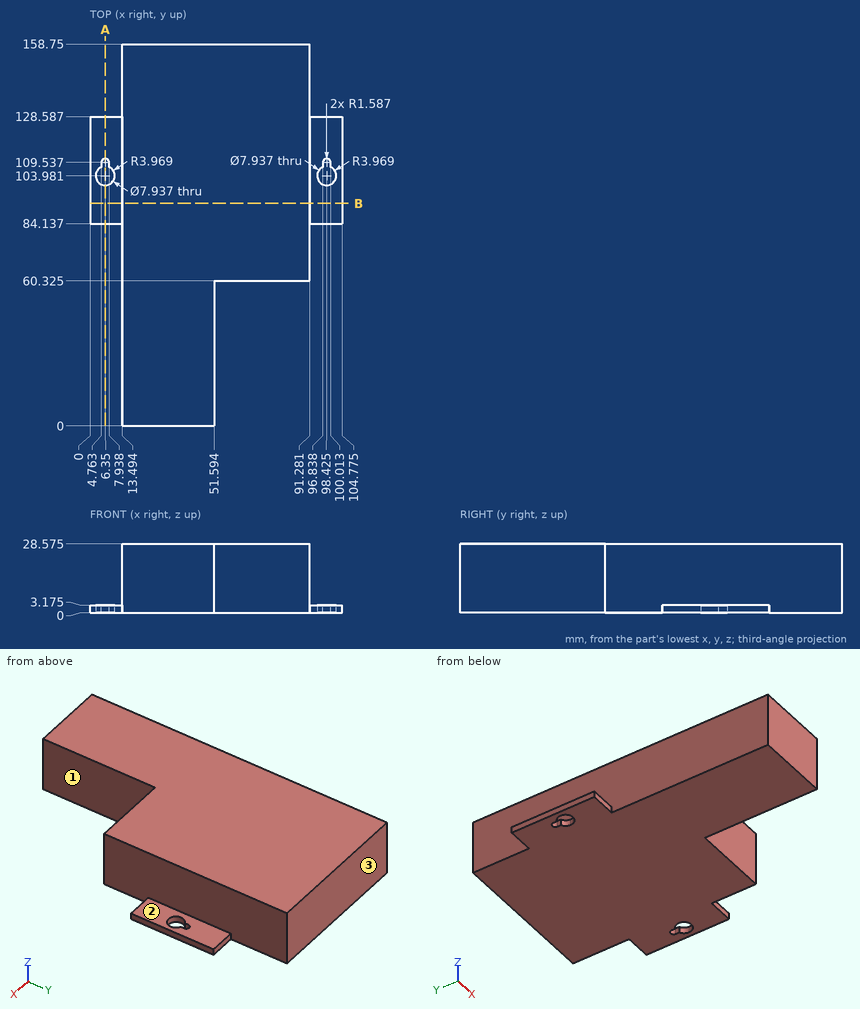
Could you check a few things on this drawing? It's one solid part, dimensions in mm from its lowest x, y, z. A direction names the side the tool comes from. Give positions to 0.01 mm unless a question says otherwise; leave off trailing zeros. Order: outer loops, then holes, each group sorted by start corner. A loop starts at its lowest first (then second) coordinate and runs counter-clockwise, first axis right, second up. Notation, with made-up numbers: (63.5, 53.25) - (115.5, 53.25) arc R13 ccw to (115.5, 62.25) - close; hole circle Ø11 at (79, -6). An arc over 180 degrees is marked (long way). Answer as a JSON object with one key per item and string values. Group by question number.
Item 1: Please list where these lines run through material, in increasing order: probe 1 along Y at (x, z) = (6.35, 1.5) (1 decimal); probe 2 along X at (y, z) = (128.5, 7.75); probe 3 along X at (y, z) = (34, 14.75).
Item 2: For P1, Ø10, axis at y = 55, z = 25, coming from the -X side; P2, Ø12.5, axis at x = 98.43, y = 103.98, coming from the +Z side (1 decimal); P3, Ø0.6, axis at y = 108, z = 2, coming from the -X side; P4, Ø1, axis at x = 96.5, z = 1.5, coming from the +Y side, each with a flat end and sliding along its axis, tell me the tip position at first contact or that it passes through.
Item 3: If we section it at A-A on x = 6.35: Please give me the cut outline in (y, z) (1 decimal), and give its area (3 significant figures).
Item 4: Which directions (+Z, -Z, +X, -X, +Y, -Y) give clear straight access to the entire face, cutting with the end or side of a thin tool? Please do the marked faces 1, 2 and 3.
Item 5: If we section it at B-B on y = 92.5: Please give me the cut outline in (x, z) (1 decimal), and give its area (3 significant figures).
Result set:
{
 "1": {"probe 1": "84.1 to 100, 111.1 to 128.6", "probe 2": "13.49 to 91.28", "probe 3": "13.49 to 51.59"},
 "2": {"P1": "x = 13.49", "P2": "z = 3.2", "P3": "x = 0", "P4": "y = 128.59"},
 "3": {"outline": "(84.1, 0) - (100, 0) - (100, 3.2) - (84.1, 3.2) - close; (111.1, 0) - (128.6, 0) - (128.6, 3.2) - (111.1, 3.2) - close", "area": "106 mm²"},
 "4": {"face 1": "+Z, -Z, +X, -Y", "face 2": "+Z, +X, +Y, -Y", "face 3": "+Z, -Z, +X, -X, +Y"},
 "5": {"outline": "(0, 0) - (104.8, 0) - (104.8, 3.2) - (91.3, 3.2) - (91.3, 28.6) - (13.5, 28.6) - (13.5, 3.2) - (0, 3.2) - close", "area": "2,310 mm²"}
}
